For this review, take the finished solid that the model builds, in its own axes (mm). A direction names the side the tool comes from. Round coordinates to 2 decimals unless told otherwise and drop trailing zeros. Write each loop counter-clockwise with the first axis right and the second up, starting at its lowest first coordinate (ties: lowest second). Pieces come first, ordered by that corner, then holes. Notation, with made-up numbers: (63.5, 5.5) -> (85.5, 5.5) arc R20 cw to (85.5, 14.5) -> close; hole circle Ø7 at (24.5, 87.5). An arc over 180 degrees is marked (long way). Answer in a Markdown table with one row per item.
from build123d import *

# Parameters (mm, degrees)
F1_DEPTH = 25.4
F2_DEPTH = 25.4
F3_DEPTH = 25.4


with BuildPart() as f1:
    # F0 (on Front) → F1 (new body)
    with BuildSketch(Plane.XZ):
        Polygon((-26.643926605, 1.6362958008), (1.6566294677, -22.7132987456), (27.8896984995, 1.0984393185), (16.8050068003, 31.0555305972), (-16.0558851046, 31.375344584), align=None)
        Polygon((-61.7250166833, 31.8198129535), (-26.643926605, 1.6362958008), (-16.0558851046, 31.375344584), align=None)
        Polygon((0, 76.4721408486), (-16.0558851046, 31.375344584), (16.8050068003, 31.0555305972), align=None)
        Polygon((16.8050068003, 31.0555305972), (27.8896984995, 1.0984393185), (60.4253225029, 30.6310020387), align=None)
        Polygon((27.8896984995, 1.0984393185), (1.6566294677, -22.7132987456), (53.0678555369, -66.9471472502), align=None)
        Polygon((-26.643926605, 1.6362958008), (-52.9653020203, -72.293587029), (1.6566294677, -22.7132987456), align=None)
    extrude(amount=F1_DEPTH)

    # F2 (add): a face of the model
    f2_faces = [f1.faces().sort_by_distance(p)[0] for p in [
        (-0.3182282883, -25.4, 0.0475680349),
    ]]
    extrude(f2_faces, amount=F2_DEPTH)

    # F3 (add): a face of the model
    f3_faces = [f1.faces().sort_by_distance(p)[0] for p in [
        (-0.3182282883, 0, 0.0475680349),
    ]]
    extrude(f3_faces, amount=F3_DEPTH)


solid = f1.part
1) Consider section C-C on z = -58. State the section outline as (x, y) points, then the cut area to 3 significant figures.
Solved:
| item | result |
|---|---|
| outline | (-47.88, -50.8) -> (-37.22, -50.8) -> (-37.22, 25.4) -> (-47.88, 25.4) -> close; (42.67, -50.8) -> (49.76, -50.8) -> (49.76, 25.4) -> (42.67, 25.4) -> close |
| area | 1,350 mm² |
2) For line 1 (X direction, y = 1, z = -51); line 2 (X direction, y = -8, z = -26); line 3 (X direction, y = -8.5, z = 38), list the stretches that pass through material, from the lowest coordinate up. Write a range as [from, to].
Solved:
| item | result |
|---|---|
| line 1 | [-45.38, -29.51], [34.53, 47.17] |
| line 2 | [-36.48, -1.96], [5.48, 37.92] |
| line 3 | [-13.7, 14.24] |
3) Consider section B-B on x = 47. State the section outline as (y, z) points.
Solved:
| item | result |
|---|---|
| outline | (-50.8, -61.73) -> (25.4, -61.73) -> (25.4, -50.55) -> (-50.8, -50.55) -> close; (-50.8, 18.44) -> (25.4, 18.44) -> (25.4, 30.76) -> (-50.8, 30.76) -> close |
4) Clearance check with flat-ended pins moving along their axes: pin 1 Ø4 at (y, z) = (11, -50) entering from -X; pin 2 Ø1.5 at (x, y) = (43, -17.5) entering from +Z; pin 3 Ø2 at (y, z) = (-6.5, -16.5) entering from -X. State where each tip first meets the part, or that it passes through.
Solved:
| item | result |
|---|---|
| pin 1 | x = -45.74 |
| pin 2 | z = 30.81 |
| pin 3 | x = -33.46 |
5) Consider section D-D on x = 24.5. State the section outline as (y, z) points, then the cut area to 3 significant figures.
Solved:
| item | result |
|---|---|
| outline | (-50.8, -42.37) -> (25.4, -42.37) -> (25.4, 30.98) -> (-50.8, 30.98) -> close |
| area | 5,590 mm² |
6) Mouldability with a two-part tool opening along Z and no side actions: class faces 1 (the flat face through (4, -50.8, 2)), 2 (the flat face through (43.93, -13.23, 15.66)), 3 (the flat face through (-26.037, -13.233, -47.851)) as pulls with the +Z half, pulls with the -Z half, needs draft (parallel to the pull), parting line crosses it, or undercut.
Solved:
| item | result |
|---|---|
| face 1 | needs draft |
| face 2 | undercut |
| face 3 | pulls with the -Z half |
7) Consider section A-A on y = -35.5. State the section outline as (x, z) points (3 decimals).
Solved:
| item | result |
|---|---|
| outline | (-61.725, 31.82) -> (-26.644, 1.636) -> (-52.965, -72.294) -> (1.657, -22.713) -> (53.068, -66.947) -> (27.89, 1.098) -> (60.425, 30.631) -> (16.805, 31.056) -> (0, 76.472) -> (-16.056, 31.375) -> close |
8) For faces 4 (the flat face through (-39.62, -13.23, -34.81)), 5 (the flat face through (27, -13.23, -44.52)), 6 (the flat face through (40.655, -13.233, -33.401)), list the 3-axis set-ups (+Z, -Z, +X, -X, +Y, -Y) from which the entire face can be reached by the end or side of a thin tool; tool diameter is ignored.
Solved:
| item | result |
|---|---|
| face 4 | -X, +Y, -Y |
| face 5 | -Z, +Y, -Y |
| face 6 | +X, +Y, -Y |
